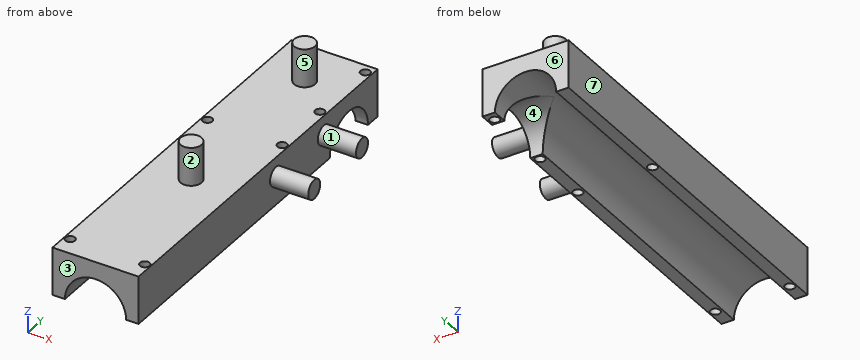
Solid Edge part; units mm, degrees
sketch "Sketch1" plane through (0, 0, 0) normal (0, -1, 0) x (1, 0, 0)
  line L0 (-22.5, -12.5) -> (22.5, -12.5)
  line L1 (22.5, -12.5) -> (22.5, 12.5)
  line L2 (-22.5, 12.5) -> (22.5, 12.5)
  line L3 (-22.5, 12.5) -> (-22.5, -12.5)
  dimension "D1" = 22.5
  dimension "D2" = 22.5
extrude "Protrusion1" add sketch "Sketch1" along normal blind 200
sketch "Sketch2" plane through (0, -200, 0) normal (0, -1, 0) x (1, 0, 0)
  line L0 (-16, -12.5) -> (16, -12.5)
  arc A0 (-16, -12.5) -> (16, -12.5) centre (0, -12.5) cw
  dimension "D1" = 16
extrude "Cutout1" cut sketch "Sketch2" against normal up to next
hole "Hole_1" at (19.5, -75, -12.5) direction (0, 0, 1) diameter 5 end up to next
hole "Hole1" at (19.5, -190, -12.5) direction (0, 0, 1) diameter 5 end up to next
hole "Hole2" at (-19.5, -190, -12.5) direction (0, 0, 1) diameter 5 end up to next
hole "Hole3" at (-19.5, -75, -12.5) direction (0, 0, 1) diameter 5 end up to next
sketch "Sketch3" plane through (22.5, -75, 0) normal (1, 0, 0) x (0, 1, 0)
  line L0 (67, -12.5) -> (35, -12.5)
  arc A0 (35, -12.5) -> (67, -12.5) centre (51, -12.5) cw
  dimension "D1" = 67
extrude "Cutout2" cut sketch "Sketch3" against normal up to next
hole "Hole_5" at (19.25, -5, -12.5) direction (0, 0, 1) diameter 5 end up to next
hole "Hole4" at (19.25, -43, -12.5) direction (0, 0, 1) diameter 5 end up to next
sketch "Sketch4" plane through (0, -100, 12.5) normal (0, 0, 1) x (0, 1, 0)
  circle A0 centre (-20, 0) radius 5.5
  circle A1 centre (75, 0) radius 5.5
extrude "ExtrudedProtrusion_2" add sketch "Sketch4" along normal blind 20
cosmetic_thread "Thread1"
cosmetic_thread "Thread2"
sketch "Sketch5" plane through (22.5, -100, 0) normal (1, 0, 0) x (0, 1, 0)
  circle A0 centre (15, 2.5) radius 5
  circle A1 centre (55, 2.5) radius 5
extrude "ExtrudedProtrusion_3" add sketch "Sketch5" along normal blind 20
cosmetic_thread "Thread3"
cosmetic_thread "Thread4"
Check sheet for the modelled part. Datum: model origin and axes. Units: mm. Face numbers are marked on the shaded views. A direction names the side the tool comes from. Coordinates: 2 decimals unless noted, no trailing zeros. Write each loop counter-clockwise with the first axis right and the second up, starting at its lowest first coordinate (ties: lowest second). Pieces come first, ordered by that corner, then holes. Notation, with made-up numbers: M 29.5,-21 L 86.5,-21 A16 cw 86.5,-7 Z; hole C 80.25,31.5 d8. An arc over 180 degrees is marked long. Write item = value, one per line. Start each with the question number.
1. Sectioned sample at B-B (z = 10). Record the cut outline in (x, y), then the cut area to 3 significant figures.
2. Sectioned sample at C-C (z = -7). State how many separate pieces and enclosed holes the cut face has, then the cut area to 3 significant figures.
3. Sectioned sample at A-A (y = -75). Record the cut outline in (x, z).
4. Go/stop test with flat-tipped pins: pin 1 (1.5 mm diameter, centred on y = -36.5, z = -2.5, fed in from +X); pin 2 (6.5 mm diameter, centred on x = 19.5, y = -75, fed in from +Z). Record where each tip stops, or that it passes through.
5. Tool access check on the marked faces 1, 2, 3 and 4. Record the directions out of +Z, -Z, +X, -X, +Y, -Y that give a thin tool (end or side, any length) a straight path to the whole face; none if there is none.
6. Thickness scan on probe 1 along Y at (x, z) = (19.5, 6); probe 2 along X at (y, z) = (-190, 5); probe 3 along Y at (x, z) = (-19.5, 1.75). Record the ranges inside material, lowest first.
7. Sectioned sample at D-D (x = 34). Record the cut outline in (y, z).
8. Mould release check, pull along Y, two halves, no side actions. Record for the marked faces 5, 6 and 7: pulls with the +Y half, pulls with the -Y half, needs draft (parallel to the pull), parting line crosses it, or undercut.
The answers:
q1.outline = M -22.5,-200 L 22.5,-200 L 22.5,0 L -22.5,0 Z; hole C -19.5,-190 d5; hole C -19.5,-75 d5; hole C 19.25,-43 d5; hole C 19.25,-5 d5; hole C 19.5,-190 d5; hole C 19.5,-75 d5
q1.area = 8,880 mm²
q2.separate_pieces = 3
q2.enclosed_holes = 6
q2.area = 2,650 mm²
q3.outline = M -22.5,-12.5 L -22,-12.5 L -22,12.5 L -22.5,12.5 Z; M -17,-12.5 L -16,-12.5 A16 cw 16,-12.5 L 17,-12.5 L 17,12.5 L -17,12.5 Z; M 22,-12.5 L 22.5,-12.5 L 22.5,12.5 L 22,12.5 Z
q4.pin_1 = 22.5
q4.pin_2 = 12.5
q5.face_1 = +X
q5.face_2 = +Z
q5.face_3 = +Z, -Z, +X, -X, -Y
q5.face_4 = -Z, +X
q6.probe_1 = -200 to -192.5, -187.5 to -77.5, -72.5 to -45.49, -40.51 to -7.49, -2.51 to 0
q6.probe_2 = -22.5 to -22, -17 to 17, 22 to 22.5
q6.probe_3 = -200 to -192.5, -187.5 to -77.5, -72.5 to 0
q7.outline = C -85,2.5 d10; C -45,2.5 d10
q8.face_5 = undercut
q8.face_6 = pulls with the +Y half
q8.face_7 = needs draft
